Here's how the part is built. I have some questions about the finished solid (model axes, mm). Face numbers are marked on the shaded views. A direction names the side the tool comes from. Coordinates: 2 decimals unless noted, no trailing zeros. Loops run counter-clockwise (first coordinate to the right, second up) from the corner with the lowest first, then second, coordinate; pieces in that order, holes last. Notation, with made-up numbers: (-26, 55) - (24, 55) arc R21 cw to (24, 68) - close; hole circle Ø2 at (46.25, 69.5). An arc over 180 degrees is marked (long way). Use a Markdown table: item, result.
```python
from build123d import *

# Parameters (mm, degrees)
F1_DEPTH = 10.4
F2_W     = 7.3
F2_H     = 20.5
F3_DEPTH = 26
F4_R     = 1.2
F5_SIZE  = 1.2


with BuildPart() as f1:
    # F0 (on Right) → F1 (new body)
    with BuildSketch(Plane.YZ):
        Polygon((0, 7.5), (0, 0), (26, 0), (26, 30), (0, 30), (0, 28), align=None)
    extrude(amount=F1_DEPTH)

    # F2 (on face) → F3 (join)
    with BuildSketch(Plane.XZ):
        with Locations((5.2, 12.25)):
            Rectangle(F2_W, F2_H)
    extrude(amount=F3_DEPTH)

    # F4
    f4_edges = [f1.edges().sort_by_distance(p)[0] for p in [
        (5.2, 26, 0),
        (5.2, 26, 30),
        (0, 26, 15),
        (10.4, 26, 15),
        (0, 13, 0),
        (10.4, 13, 0),
        (0, 13, 30),
        (10.4, 13, 30),
    ]]
    fillet(f4_edges, radius=F4_R)

    # F5
    f5_edges = [f1.edges().sort_by_distance(p)[0] for p in [
        (1.55, -26, 12.25),
        (8.85, -26, 12.25),
        (8.85, -13, 22.5),
        (1.55, -13, 22.5),
        (5.2, -26, 22.5),
        (5.2, -26, 2),
    ]]
    chamfer(f5_edges, length=F5_SIZE)


solid = f1.part
```
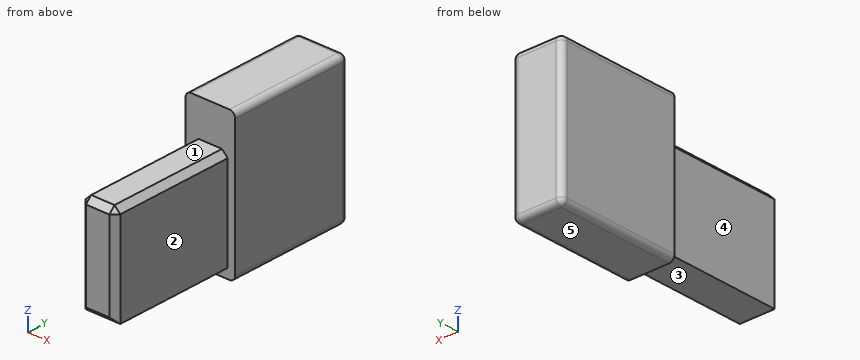
Q1. I want a section at C-C, the plane y = -2.5. Write out the boundary of the cut face in (x, z), then the cut area to 3 significant figures.
Check values:
| item | result |
|---|---|
| outline | (1.55, 2) - (8.85, 2) - (8.85, 21.3) - (7.65, 22.5) - (2.75, 22.5) - (1.55, 21.3) - close |
| area | 148 mm^2 |
Q2. Please list where these lines run through material, in increasing order: L1, parallel to X at y = -21.5, z = 11.75; L2, parallel to Y at x = 1.5, z = 9; L3, parallel to Z at x = 2.5, y = -18.5. Write a range as from..to.
Check values:
| item | result |
|---|---|
| L1 | 1.55..8.85 |
| L2 | 0..26 |
| L3 | 2..22.25 |
Q3. I want a section at A-A, the plane z = 14.5. Write out the boundary of the cut face in (x, y), then the cut area to 3 significant figures.
Check values:
| item | result |
|---|---|
| outline | (0, 0) - (1.55, 0) - (1.55, -24.8) - (2.75, -26) - (7.65, -26) - (8.85, -24.8) - (8.85, 0) - (10.4, 0) - (10.4, 24.8) arc R1.2 ccw to (9.2, 26) - (1.2, 26) arc R1.2 ccw to (0, 24.8) - close |
| area | 458 mm^2 |
Q4. I want a section at D-D, the plane x = 9.75. Write out the boundary of the cut face in (y, z), then the cut area to 3 significant figures.
Check values:
| item | result |
|---|---|
| outline | (0, 0.13) - (24.8, 0.13) arc R1.07 ccw to (25.87, 1.2) - (25.87, 28.8) arc R1.07 ccw to (24.8, 29.87) - (0, 29.87) - close |
| area | 769 mm^2 |
Q5. I want a section at B-B, the plane x = 4.5. Write out the boundary of the cut face in (y, z).
Check values:
| item | result |
|---|---|
| outline | (-26, 3.2) - (-24.8, 2) - (0, 2) - (0, 0) - (24.8, 0) arc R1.2 ccw to (26, 1.2) - (26, 28.8) arc R1.2 ccw to (24.8, 30) - (0, 30) - (0, 22.5) - (-24.8, 22.5) - (-26, 21.3) - close |
Q6. Which directions (+Z, -Z, +X, -X, +Y, -Y) give clear straight access to the entire face, cutting with the end or side of a thin tool? Please do the marked faces 1, 2, 3, 4 and 5.
Check values:
| item | result |
|---|---|
| face 1 | +Z, +X, -X, -Y |
| face 2 | +Z, -Z, +X, -Y |
| face 3 | -Z, +X, -X, -Y |
| face 4 | +Z, -Z, -X, -Y |
| face 5 | -Z, +X, -X, +Y, -Y |
Q7. Will these pins go through, and if not, where does the flat tip stop? P1, Ø2, axis at x = 2.5, y = -19.5, coming from the +Z side; P2, Ø6, axis at y = -15.5, z = 14.5, coming from the -X side; P3, Ø3.5, axis at x = 6, y = -15, coming from the -Z side.
Check values:
| item | result |
|---|---|
| P1 | z = 22.5 |
| P2 | x = 1.55 |
| P3 | z = 2 |
